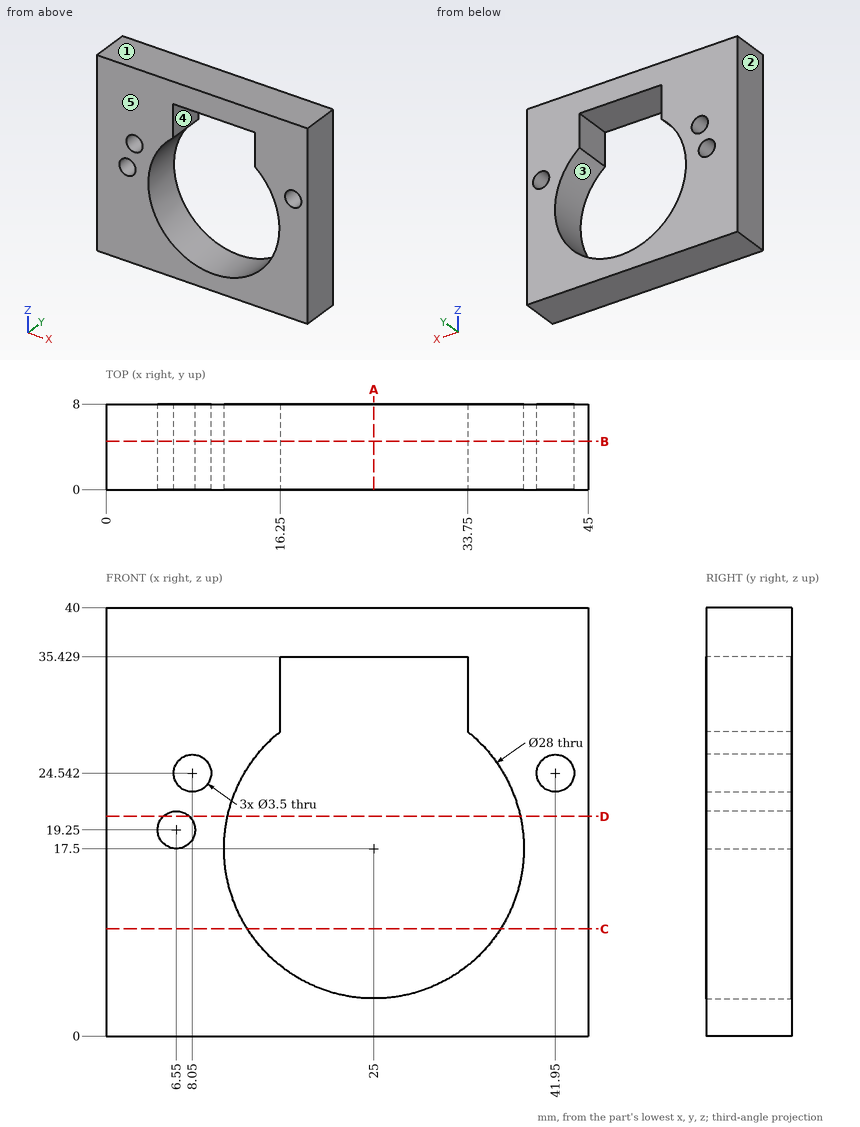
Design review of the part shown in the three views and the two pictorial views. Dimensions are in mm from the part's minimum x, y and z. A direction names the side the tool comes from. Round coordinates to 2 decimals unless told otherwise and drop trailing zeros. Write each loop counter-clockwise with the first axis right and the second up, starting at its lowest first coordinate (ties: lowest second). Pieces come first, ordered by that corner, then holes. Notation, with made-up numbers: M 86,-26 L 106,-26 A27 cw 106,8 Z; hole C 68,1.25 d6. An arc over 180 degrees is marked long. One line per item, written item: value. Start each with the question number.
1. To check wall thickness, follow probe 1 along X at (y, z) = (6.25, 19.25); probe 2 along X at (y, z) = (1.5, 24) (1 decimal); probe 3 along Z at (x, y) = (25, 3). State the ranges of each line that lie inside material, in increasing order. Write a range as from..to.
2. For the marked faces 4 and 5, list the 3-axis set-ups (+Z, -Z, +X, -X, +Y, -Y) from which the entire face can be reached by the end or side of a thin tool; tool diameter is ignored.
3. Take a section at C-C on z = 10. State the section outline as (x, y) points.
4. Take a section at D-D on z = 20.5. State the section outline as (x, y) points (1 decimal), then the cut area to 3 significant figures.
5. Take a section at A-A on x = 25. State the section outline as (y, z) points.
6. Clearance check with flat-ended pins moving along their axes: P1, Ø10, axis at x = 33.5, z = 20, coming from the +Y side; P2, Ø4, axis at y = 4.5, z = 21, coming from the -X side. State where each tip first meets the part, or that it passes through.
7. Take a section at B-B on y = 4.5. State the section outline as (x, z) points.
8. Draft analysis for pull direction X (two halves, no side actions). For the marked faces 1, 2 and 3, state which applies: pulls with the +X half, pulls with the -X half, needs draft (parallel to the pull), parting line crosses it, or undercut.
Computed:
1. probe 1: x = 0..4.8, 8.3..11.11, 38.89..45
1. probe 2: x = 0..6.4, 9.7..12.6, 37.4..40.3, 43.6..45
1. probe 3: z = 0..3.5, 35.43..40
2. face 4: +Y, -Y
2. face 5: +Z, -Z, +X, -X, -Y
3. outline: M 0,0 L 13.18,0 L 13.18,8 L 0,8 Z; M 36.82,0 L 45,0 L 45,8 L 36.82,8 Z
4. outline: M 0,0 L 5.3,0 L 5.3,8 L 0,8 Z; M 7.8,0 L 11.3,0 L 11.3,8 L 7.8,8 Z; M 38.7,0 L 45,0 L 45,8 L 38.7,8 Z
4. area: 122 mm²
5. outline: M 0,0 L 8,0 L 8,3.5 L 0,3.5 Z; M 0,35.43 L 8,35.43 L 8,40 L 0,40 Z
6. P1: passes through
6. P2: stops at x = 0
7. outline: M 0,0 L 45,0 L 45,40 L 0,40 Z; hole C 6.55,19.25 d3.5; hole C 8.05,24.54 d3.5; hole M 16.25,28.43 A14 ccw long 33.75,28.43 L 33.75,35.43 L 16.25,35.43 Z; hole C 41.95,24.54 d3.5
8. face 1: needs draft
8. face 2: pulls with the -X half
8. face 3: undercut
